Geometry: final body of the model. Coordinates: model frame, mm. A direction names the side the tool comes from. Coordinates: 2 decimals unless noted, no trailing zeros. Write each loop counter-clockwise with the first axis right and the second up, starting at its lowest first coordinate (ties: lowest second). Pieces come first, ordered by that corner, then holes.
from build123d import *

# Parameters (mm, degrees)
BOSS_EXTRUDE1_DEPTH = 0.8
SKETCH2_W           = 100.7
SKETCH2_H           = 166.5
BOSS_EXTRUDE2_DEPTH = 5.3
SKETCH3_W           = 7.8
SKETCH3_H           = 15
SKETCH3_R           = 1.5
BOSS_EXTRUDE3_DEPTH = 2.6
SKETCH4_W           = 58.5
SKETCH4_H           = 90.5
BOSS_EXTRUDE4_DEPTH = 34
CHAMFER1_SIZE       = 3


with BuildPart() as part:
    # Sketch1 → Boss-Extrude1 (new body)
    with BuildSketch(Plane.XY):
        with BuildLine():
            Line((47.4, -96.5), (-47.4, -96.5))
            ThreePointArc((-47.4, -96.5), (-53.056854249, -94.156854249), (-55.4, -88.5))
            Line((-55.4, -88.5), (-55.4, 88.5))
            ThreePointArc((-55.4, 88.5), (-53.056854249, 94.156854249), (-47.4, 96.5))
            Line((-47.4, 96.5), (47.4, 96.5))
            ThreePointArc((47.4, 96.5), (53.056854249, 94.156854249), (55.4, 88.5))
            Line((55.4, 88.5), (55.4, -88.5))
            ThreePointArc((55.4, -88.5), (53.056854249, -94.156854249), (47.4, -96.5))
        make_face()
    extrude(amount=-BOSS_EXTRUDE1_DEPTH)

    # Sketch2 → Boss-Extrude2 (add)
    with BuildSketch(Plane(origin=(0, 0, -0.8), x_dir=(-1, 0, 0), z_dir=(0, 0, -1))):
        with Locations((1.4, -1.6)):
            Rectangle(SKETCH2_W, SKETCH2_H)
    extrude(amount=BOSS_EXTRUDE2_DEPTH)

    # Sketch3 → Boss-Extrude3 (add)
    # profile 1 of 4: a face of its own
    with BuildSketch(Plane(origin=(0, 0, -6.1), x_dir=(-1, 0, 0), z_dir=(0, 0, -1))):
        with Locations((-34.05, 61.65)):
            Rectangle(SKETCH3_W, SKETCH3_H)
        with Locations((-34.05, 61.65)):
            Circle(SKETCH3_R, mode=Mode.SUBTRACT)
    # profile 2 of 4: a face of its own
    with BuildSketch(Plane(origin=(0, 0, -6.1), x_dir=(-1, 0, 0), z_dir=(0, 0, -1))):
        with Locations((31.65, 61.65)):
            Rectangle(SKETCH3_W, SKETCH3_H)
        with Locations((31.65, 61.65)):
            Circle(SKETCH3_R, mode=Mode.SUBTRACT)
    # profile 3 of 4: a face of its own
    with BuildSketch(Plane(origin=(0, 0, -6.1), x_dir=(-1, 0, 0), z_dir=(0, 0, -1))):
        with Locations((-34.05, -64.55)):
            Rectangle(SKETCH3_W, SKETCH3_H)
        with Locations((-34.05, -64.55)):
            Circle(SKETCH3_R, mode=Mode.SUBTRACT)
    # profile 4 of 4: a face of its own
    with BuildSketch(Plane(origin=(0, 0, -6.1), x_dir=(-1, 0, 0), z_dir=(0, 0, -1))):
        with Locations((31.65, -64.55)):
            Rectangle(SKETCH3_W, SKETCH3_H)
        with Locations((31.65, -64.55)):
            Circle(SKETCH3_R, mode=Mode.SUBTRACT)
    extrude(amount=BOSS_EXTRUDE3_DEPTH)

    # Sketch4 → Boss-Extrude4 (add)
    with BuildSketch(Plane(origin=(0, 0, -6.1), x_dir=(-1, 0, 0), z_dir=(0, 0, -1))):
        with Locations((-2.5, 3.4)):
            Rectangle(SKETCH4_W, SKETCH4_H)
    extrude(amount=BOSS_EXTRUDE4_DEPTH)

    # Chamfer1
    # the kernel refuses this chamfer: 3 mm, written as the material it takes off along each edge
    with BuildSketch(Plane(origin=(-20.034951036, -72.05, -8.7), x_dir=(0, -0.027495876610586775, 0.9996219169112968), z_dir=(-1, 0, 0))) as chamfer1_piece_1_section:
        Polygon((CHAMFER1_SIZE * 0.999621916911, CHAMFER1_SIZE * 0.0274958766106), (-CHAMFER1_SIZE * 0.0274958766106, CHAMFER1_SIZE * 0.999621916911), (0, 0), align=None)
    chamfer1_piece_1 = extrude(amount=23.230097928, mode=Mode.PRIVATE)
    chamfer1_piece_1 = split(chamfer1_piece_1, bisect_by=Plane(origin=(-31.65, -71.03377063, -6.1), z_dir=(0, 0, -1)), keep=Keep.TOP, mode=Mode.PRIVATE)
    add(chamfer1_piece_1, mode=Mode.SUBTRACT)
    with BuildSketch(Plane(origin=(-43.265048964, -57.05, -8.7), x_dir=(0, 0.027495876610586775, 0.9996219169112968), z_dir=(1, 0, 0))) as chamfer1_piece_2_section:
        Polygon((CHAMFER1_SIZE * 0.999621916911, CHAMFER1_SIZE * 0.0274958766106), (-CHAMFER1_SIZE * 0.0274958766106, CHAMFER1_SIZE * 0.999621916911), (0, 0), align=None)
    chamfer1_piece_2 = extrude(amount=23.230097928, mode=Mode.PRIVATE)
    chamfer1_piece_2 = split(chamfer1_piece_2, bisect_by=Plane(origin=(-31.65, -58.06622937, -6.1), z_dir=(0, 0, -1)), keep=Keep.TOP, mode=Mode.PRIVATE)
    add(chamfer1_piece_2, mode=Mode.SUBTRACT)
    with BuildSketch(Plane(origin=(22.434951036, -72.05, -8.7), x_dir=(0, -0.027495876610586775, 0.9996219169112968), z_dir=(1, 0, 0))) as chamfer1_piece_3_section:
        Polygon((CHAMFER1_SIZE * 0.999621916911, -CHAMFER1_SIZE * 0.0274958766106), (-CHAMFER1_SIZE * 0.0274958766106, -CHAMFER1_SIZE * 0.999621916911), (0, 0), align=None)
    chamfer1_piece_3 = extrude(amount=23.230097928, mode=Mode.PRIVATE)
    chamfer1_piece_3 = split(chamfer1_piece_3, bisect_by=Plane(origin=(34.05, -71.03377063, -6.1), z_dir=(0, 0, -1)), keep=Keep.TOP, mode=Mode.PRIVATE)
    add(chamfer1_piece_3, mode=Mode.SUBTRACT)
    with BuildSketch(Plane(origin=(45.665048964, -57.05, -8.7), x_dir=(0, 0.027495876610586775, 0.9996219169112968), z_dir=(-1, 0, 0))) as chamfer1_piece_4_section:
        Polygon((CHAMFER1_SIZE * 0.999621916911, -CHAMFER1_SIZE * 0.0274958766106), (-CHAMFER1_SIZE * 0.0274958766106, -CHAMFER1_SIZE * 0.999621916911), (0, 0), align=None)
    chamfer1_piece_4 = extrude(amount=23.230097928, mode=Mode.PRIVATE)
    chamfer1_piece_4 = split(chamfer1_piece_4, bisect_by=Plane(origin=(34.05, -58.06622937, -6.1), z_dir=(0, 0, -1)), keep=Keep.TOP, mode=Mode.PRIVATE)
    add(chamfer1_piece_4, mode=Mode.SUBTRACT)
    with BuildSketch(Plane(origin=(45.665048964, 54.15, -8.7), x_dir=(0, -0.027495876610586775, 0.9996219169112968), z_dir=(-1, 0, 0))) as chamfer1_piece_5_section:
        Polygon((CHAMFER1_SIZE * 0.999621916911, CHAMFER1_SIZE * 0.0274958766106), (-CHAMFER1_SIZE * 0.0274958766106, CHAMFER1_SIZE * 0.999621916911), (0, 0), align=None)
    chamfer1_piece_5 = extrude(amount=23.230097928, mode=Mode.PRIVATE)
    chamfer1_piece_5 = split(chamfer1_piece_5, bisect_by=Plane(origin=(34.05, 55.16622937, -6.1), z_dir=(0, 0, -1)), keep=Keep.TOP, mode=Mode.PRIVATE)
    add(chamfer1_piece_5, mode=Mode.SUBTRACT)
    with BuildSketch(Plane(origin=(22.434951036, 69.15, -8.7), x_dir=(0, 0.027495876610586775, 0.9996219169112968), z_dir=(1, 0, 0))) as chamfer1_piece_6_section:
        Polygon((CHAMFER1_SIZE * 0.999621916911, CHAMFER1_SIZE * 0.0274958766106), (-CHAMFER1_SIZE * 0.0274958766106, CHAMFER1_SIZE * 0.999621916911), (0, 0), align=None)
    chamfer1_piece_6 = extrude(amount=23.230097928, mode=Mode.PRIVATE)
    chamfer1_piece_6 = split(chamfer1_piece_6, bisect_by=Plane(origin=(34.05, 68.13377063, -6.1), z_dir=(0, 0, -1)), keep=Keep.TOP, mode=Mode.PRIVATE)
    add(chamfer1_piece_6, mode=Mode.SUBTRACT)
    with BuildSketch(Plane(origin=(-43.265048964, 54.15, -8.7), x_dir=(0, -0.027495876610586775, 0.9996219169112968), z_dir=(1, 0, 0))) as chamfer1_piece_7_section:
        Polygon((CHAMFER1_SIZE * 0.999621916911, -CHAMFER1_SIZE * 0.0274958766106), (-CHAMFER1_SIZE * 0.0274958766106, -CHAMFER1_SIZE * 0.999621916911), (0, 0), align=None)
    chamfer1_piece_7 = extrude(amount=23.230097928, mode=Mode.PRIVATE)
    chamfer1_piece_7 = split(chamfer1_piece_7, bisect_by=Plane(origin=(-31.65, 55.16622937, -6.1), z_dir=(0, 0, -1)), keep=Keep.TOP, mode=Mode.PRIVATE)
    add(chamfer1_piece_7, mode=Mode.SUBTRACT)
    with BuildSketch(Plane(origin=(-20.034951036, 69.15, -8.7), x_dir=(0, 0.027495876610586775, 0.9996219169112968), z_dir=(-1, 0, 0))) as chamfer1_piece_8_section:
        Polygon((CHAMFER1_SIZE * 0.999621916911, -CHAMFER1_SIZE * 0.0274958766106), (-CHAMFER1_SIZE * 0.0274958766106, -CHAMFER1_SIZE * 0.999621916911), (0, 0), align=None)
    chamfer1_piece_8 = extrude(amount=23.230097928, mode=Mode.PRIVATE)
    chamfer1_piece_8 = split(chamfer1_piece_8, bisect_by=Plane(origin=(-31.65, 68.13377063, -6.1), z_dir=(0, 0, -1)), keep=Keep.TOP, mode=Mode.PRIVATE)
    add(chamfer1_piece_8, mode=Mode.SUBTRACT)


solid = part.part
Item 1: Pin query (flat end, axial travel): pin 1 (8.5 mm diameter, centred on x = 32, y = 61.5, fed in from -Z); pin 2 (12 mm diameter, centred on y = -20.5, z = -15, fed in from -X); pin 3 (2.5 mm diameter, centred on x = 34.05, y = -64.55, fed in from -Z). Return the tip coordinate at first contact, or that it passes through.
Derived:
pin 1: stops at z = -8.7
pin 2: stops at x = -26.75
pin 3: stops at z = -6.1
Item 2: Material intervals for probe 1 along X at (y, z) = (-64.55, -7.8); probe 2 along Y at (x, z) = (-31.65, -7.9); probe 3 along Y at (x, z) = (34, -7), sorted ascending.
Derived:
probe 1: x = -35.55 to -33.15, -30.15 to -27.75, 30.15 to 32.55, 35.55 to 37.95
probe 2: y = -69.85 to -66.05, -63.05 to -59.25, 56.35 to 60.15, 63.15 to 66.95
probe 3: y = -70.75 to -66.05, -63.05 to -58.35, 55.45 to 60.15, 63.15 to 67.85
Item 3: Section B-B, the plane x = 8. Output: boundary loops of the cut face in (y, z).
Derived:
outline: (-96.5, -0.8) - (-84.85, -0.8) - (-84.85, -6.1) - (-41.85, -6.1) - (-41.85, -40.1) - (48.65, -40.1) - (48.65, -6.1) - (81.65, -6.1) - (81.65, -0.8) - (96.5, -0.8) - (96.5, 0) - (-96.5, 0) - close
Item 4: Set-up query: faces 1 (the flat face through (-1, 81.65, -3)), 2 (the flat face through (-33.3, 61.7, -8.7)), 3 (the flat face through (36, -64, -8.7)), 4 (the flat face through (-51.75, -3, -3)), 5 (the flat face through (48.95, -3, -3)). Return all of +Z, -Z, +X, -X, +Y, -Y with unobstructed straight access to the full face (end or side cutting, diameter ignored); none if empty.
Derived:
face 1: -Z, +X, -X, +Y
face 2: -Z, +X, -X, +Y, -Y
face 3: -Z, +X, -X, -Y
face 4: -Z, -X, +Y, -Y
face 5: -Z, +X, +Y, -Y
Item 5: Section A-A, the plane y = 5. Output: boundary loops of the cut face in (x, z).
Derived:
outline: (-55.4, -0.8) - (-51.75, -0.8) - (-51.75, -6.1) - (-26.75, -6.1) - (-26.75, -40.1) - (31.75, -40.1) - (31.75, -6.1) - (48.95, -6.1) - (48.95, -0.8) - (55.4, -0.8) - (55.4, 0) - (-55.4, 0) - close
Item 6: Section C-C, the plane z = -26.5. Output: boundary loops of the cut face in (x, y), plus the area to 3 significant figures.
Derived:
outline: (-26.75, -41.85) - (31.75, -41.85) - (31.75, 48.65) - (-26.75, 48.65) - close
area: 5,290 mm2
Item 7: Section D-D, the plane y = -50. Output: boundary loops of the cut face in (x, z).
Derived:
outline: (-55.4, -0.8) - (-51.75, -0.8) - (-51.75, -6.1) - (48.95, -6.1) - (48.95, -0.8) - (55.4, -0.8) - (55.4, 0) - (-55.4, 0) - close
Item 8: Pull-direction query (X, two-part tool) for faces 6 (the flat face through (-26.75, 3, -23)), 7 (the cylindrical face through (52.994, 94.219, -0.394)), 8 (the flat face through (3, -41.85, -23)); classes: released by +X, released by -X, zero draft, split by the parting line, or undercut.
Derived:
face 6: released by -X
face 7: released by +X
face 8: zero draft
